Design review of the part built by this model. Coordinates are the model's own, in mm. Give positions to 0.01 mm unless a question says otherwise; leave off trailing zeros. Loops run counter-clockwise (first coordinate to the right, second up) from the corner with the lowest first, then second, coordinate; pieces in that order, holes last. Notation, with made-up numbers: M 14.25,72.5 L 19.25,72.5 A13 ccw 19.25,93.5 Z; hole C 19.25,-14.75 d2. An arc over 180 degrees is marked long. Use a Markdown table: item, result. Add a question column.
(1) Add section C-C, the plane z = -23.5. Give the boundary of the cut face in (x, y), then the cut area to 3 significant figures.
(2) For probe 1 along Z at (x, y) = (0, 1.1); probe 2 along X at (y, z) = (0.6, -21); probe 3 along X at (y, z) = (1.05, -11), list the stretches that pass through material, from the lowest coordinate up.
(3) Add section B-B, the plane y = 1.1. Give the boundary of the cut face in (x, z).
(4) Insertion check: pin 1 Ø6 at (x, z) = (-40, 0) entering from -Y. The pin has a flat end and moves straight along its axis. Give the tip position at first contact, or say it passes through.
(5) Add section A-A, the plane x = 0. Give the boundary of the cut face in (y, z).
(6) Add section D-D, the plane x = 40. Give the boundary of the cut face in (y, z).
Autodesk Inventor part; units mm, degrees
ref_plane "YZ Plane" through (0, 0, 0) normal (1, 0, 0) x (0, 1, 0)
ref_plane "XZ Plane" through (0, 0, 0) normal (0, 1, 0) x (-1, 0, 0)
ref_plane "XY Plane" through (0, 0, 0) normal (0, 0, 1) x (1, 0, 0)
sketch "Sketch1" plane through (0, 0, 0) normal (0, 1, 0) x (-1, 0, 0)
  circle A0 centre (0, 0) radius 52.7 construction
  circle A1 centre (0, 0) radius 55 construction
  circle A2 centre (0, 0) radius 57 construction
  circle A3 centre (0, 0) radius 30
  circle A4 centre (0, 0) radius 46.5
  circle A5 centre (0, 0) radius 40 construction
  circle A6 centre (40, 0) radius 3.75
  circle A7 centre (0, -40) radius 3.75
  circle A8 centre (-40, 0) radius 3.75
  circle A9 centre (0, 40) radius 3.75
  dimension "d0" = 105.4
  dimension "d1" = 110
  dimension "d2" = 114
  dimension "d3" = 60
  dimension "d4" = 93
  dimension "d5" = 80
  dimension "d6" = 7.5
  dimension "d7" = 7.5
  dimension "d8" = 7.5
  dimension "d9" = 7.5
extrude "Extrusion1" add sketch "Sketch1" along normal blind 2
properties part number "BiggerFanFlange"
Established:
| question | item | result |
|---|---|---|
| 1 | outline | M -40.12,0 L -18.65,0 L -18.65,2 L -40.12,2 Z; M 18.65,0 L 40.12,0 L 40.12,2 L 18.65,2 Z |
| 1 | area | 85.9 mm^2 |
| 2 | probe 1 | -46.5 to -43.75, -36.25 to -30, 30 to 36.25, 43.75 to 46.5 |
| 2 | probe 2 | -41.49 to -21.42, 21.42 to 41.49 |
| 2 | probe 3 | -45.18 to -27.91, 27.91 to 45.18 |
| 3 | outline | C 0,0 d93; hole C -40,0 d7.5; hole C 0,0 d60; hole C 0,-40 d7.5; hole C 0,40 d7.5; hole C 40,0 d7.5 |
| 4 | pin 1 | through |
| 5 | outline | M 0,-46.5 L 2,-46.5 L 2,-43.75 L 0,-43.75 Z; M 0,-36.25 L 2,-36.25 L 2,-30 L 0,-30 Z; M 0,30 L 2,30 L 2,36.25 L 0,36.25 Z; M 0,43.75 L 2,43.75 L 2,46.5 L 0,46.5 Z |
| 6 | outline | M 0,-23.71 L 2,-23.71 L 2,-3.75 L 0,-3.75 Z; M 0,3.75 L 2,3.75 L 2,23.71 L 0,23.71 Z |
